from build123d import *

# Parameters (mm, degrees)
F0_W     = 75
F0_H     = 75
F0_R     = 3.75
F1_DEPTH = 2
F2_DEPTH = 16
F3_W     = 75
F3_H     = 75
F3_R     = 3.75
F3_W_2   = 50
F3_H_2   = 50
F4_DEPTH = 6.5
F5_W     = 1
F5_H     = 1
F6_DEPTH = 1


with BuildPart() as f1:
    # F0 (on Top) → F1 (new body)
    with BuildSketch(Plane.XY):
        Rectangle(F0_W, F0_H)
        with Locations((-31.25, -31.25)):
            Circle(F0_R, mode=Mode.SUBTRACT)
        with Locations((31.25, -31.25)):
            Circle(F0_R, mode=Mode.SUBTRACT)
        with Locations((-31.25, 31.25)):
            Circle(F0_R, mode=Mode.SUBTRACT)
        with Locations((31.25, 31.25)):
            Circle(F0_R, mode=Mode.SUBTRACT)
        with Locations((-31.25, 31.25)):
            Circle(F0_R)
        with Locations((31.25, 31.25)):
            Circle(F0_R)
        with Locations((31.25, -31.25)):
            Circle(F0_R)
        with Locations((-31.25, -31.25)):
            Circle(F0_R)
    extrude(amount=F1_DEPTH)

    # F0 (on Top) → F2 (join)
    with BuildSketch(Plane.XY):
        with Locations((-31.25, -31.25)):
            Circle(F0_R)
        with Locations((31.25, -31.25)):
            Circle(F0_R)
        with Locations((-31.25, 31.25)):
            Circle(F0_R)
        with Locations((31.25, 31.25)):
            Circle(F0_R)
    extrude(amount=F2_DEPTH)

    # F3 (on face) → F4 (join)
    with BuildSketch(Plane.XY.offset(2)):
        Rectangle(F3_W, F3_H)
        with Locations((-31.25, -31.25)):
            Circle(F3_R, mode=Mode.SUBTRACT)
        with Locations((31.25, -31.25)):
            Circle(F3_R, mode=Mode.SUBTRACT)
        with Locations((-31.25, 31.25)):
            Circle(F3_R, mode=Mode.SUBTRACT)
        Rectangle(F3_W_2, F3_H_2, mode=Mode.SUBTRACT)
        with Locations((31.25, 31.25)):
            Circle(F3_R, mode=Mode.SUBTRACT)
    extrude(amount=F4_DEPTH)

    # F5 (on face) → F6 (cut)
    with BuildSketch(Plane.XY):
        with BuildLine():
            Line((-32.5, -34.7855339059), (-32.5, -37.5))
            Line((-32.5, -37.5), (-31.5, -37.5))
            Line((-31.5, -37.5), (-31.5, -34.9916573868))
            ThreePointArc((-31.5, -34.9916573868), (-32.0070480317, -34.9227888964), (-32.5, -34.7855339059))
        make_face()
        with BuildLine():
            Line((-32.5, -32.5), (-32.5, -34.7855339059))
            ThreePointArc((-32.5, -34.7855339059), (-32.0070480317, -34.9227888964), (-31.5, -34.9916573868))
            Line((-31.5, -34.9916573868), (-31.5, -32.5))
            Line((-31.5, -32.5), (-32.5, -32.5))
        make_face()
        with BuildLine():
            Line((31.5, -34.9916573868), (31.5, -37.5))
            Line((31.5, -37.5), (32.5, -37.5))
            Line((32.5, -37.5), (32.5, -34.7855339059))
            ThreePointArc((32.5, -34.7855339059), (32.0070480317, -34.9227888964), (31.5, -34.9916573868))
        make_face()
        with BuildLine():
            Line((-34.7855339059, -32.5), (-32.5, -32.5))
            Line((-32.5, -32.5), (-32.5, -31.5))
            Line((-32.5, -31.5), (-34.9916573868, -31.5))
            ThreePointArc((-34.9916573868, -31.5), (-34.9227888964, -32.0070480317), (-34.7855339059, -32.5))
        make_face()
        with Locations((-32, -32)):
            Rectangle(F5_W, F5_H)
        with BuildLine():
            Line((-37.5, -32.5), (-34.7855339059, -32.5))
            ThreePointArc((-34.7855339059, -32.5), (-34.9227888964, -32.0070480317), (-34.9916573868, -31.5))
            Line((-34.9916573868, -31.5), (-37.5, -31.5))
            Line((-37.5, -31.5), (-37.5, -32.5))
        make_face()
        with BuildLine():
            Line((-31.5, -31.5), (-31.5, -32.5))
            Line((-31.5, -32.5), (-27.7144660941, -32.5))
            ThreePointArc((-27.7144660941, -32.5), (-27.5772111036, -32.0070480317), (-27.5083426132, -31.5))
            Line((-27.5083426132, -31.5), (-31.5, -31.5))
        make_face()
        with BuildLine():
            ThreePointArc((-27.5083426132, -31.5), (-27.5772111036, -32.0070480317), (-27.7144660941, -32.5))
            Line((-27.7144660941, -32.5), (27.7144660941, -32.5))
            ThreePointArc((27.7144660941, -32.5), (27.5772111036, -32.0070480317), (27.5083426132, -31.5))
            Line((27.5083426132, -31.5), (-27.5083426132, -31.5))
        make_face()
        with BuildLine():
            Line((31.5, -32.5), (31.5, -34.9916573868))
            ThreePointArc((31.5, -34.9916573868), (32.0070480317, -34.9227888964), (32.5, -34.7855339059))
            Line((32.5, -34.7855339059), (32.5, -32.5))
            Line((32.5, -32.5), (31.5, -32.5))
        make_face()
        with BuildLine():
            Line((-32.5, -27.7144660941), (-32.5, -31.5))
            Line((-32.5, -31.5), (-31.5, -31.5))
            Line((-31.5, -31.5), (-31.5, -27.5083426132))
            ThreePointArc((-31.5, -27.5083426132), (-32.0070480317, -27.5772111036), (-32.5, -27.7144660941))
        make_face()
        with BuildLine():
            ThreePointArc((27.5083426132, -31.5), (27.5772111036, -32.0070480317), (27.7144660941, -32.5))
            Line((27.7144660941, -32.5), (31.5, -32.5))
            Line((31.5, -32.5), (31.5, -31.5))
            Line((31.5, -31.5), (27.5083426132, -31.5))
        make_face()
        with Locations((32, -32)):
            Rectangle(F5_W, F5_H)
        with BuildLine():
            Line((-32.5, 27.7144660941), (-32.5, -27.7144660941))
            ThreePointArc((-32.5, -27.7144660941), (-32.0070480317, -27.5772111036), (-31.5, -27.5083426132))
            Line((-31.5, -27.5083426132), (-31.5, 27.5083426132))
            ThreePointArc((-31.5, 27.5083426132), (-32.0070480317, 27.5772111036), (-32.5, 27.7144660941))
        make_face()
        with BuildLine():
            Line((-37.5, 32.5), (-37.5, 31.5))
            Line((-37.5, 31.5), (-34.9916573868, 31.5))
            ThreePointArc((-34.9916573868, 31.5), (-34.9227888964, 32.0070480317), (-34.7855339059, 32.5))
            Line((-34.7855339059, 32.5), (-37.5, 32.5))
        make_face()
        with BuildLine():
            Line((32.5, -31.5), (32.5, -32.5))
            Line((32.5, -32.5), (34.7855339059, -32.5))
            ThreePointArc((34.7855339059, -32.5), (34.9227888964, -32.0070480317), (34.9916573868, -31.5))
            Line((34.9916573868, -31.5), (32.5, -31.5))
        make_face()
        with BuildLine():
            ThreePointArc((34.9916573868, -31.5), (34.9227888964, -32.0070480317), (34.7855339059, -32.5))
            Line((34.7855339059, -32.5), (37.5, -32.5))
            Line((37.5, -32.5), (37.5, -31.5))
            Line((37.5, -31.5), (34.9916573868, -31.5))
        make_face()
        with BuildLine():
            Line((31.5, -27.5083426132), (31.5, -31.5))
            Line((31.5, -31.5), (32.5, -31.5))
            Line((32.5, -31.5), (32.5, -27.7144660941))
            ThreePointArc((32.5, -27.7144660941), (32.0070480317, -27.5772111036), (31.5, -27.5083426132))
        make_face()
        with BuildLine():
            Line((-32.5, 31.5), (-32.5, 27.7144660941))
            ThreePointArc((-32.5, 27.7144660941), (-32.0070480317, 27.5772111036), (-31.5, 27.5083426132))
            Line((-31.5, 27.5083426132), (-31.5, 31.5))
            Line((-31.5, 31.5), (-32.5, 31.5))
        make_face()
        with BuildLine():
            ThreePointArc((-34.7855339059, 32.5), (-34.9227888964, 32.0070480317), (-34.9916573868, 31.5))
            Line((-34.9916573868, 31.5), (-32.5, 31.5))
            Line((-32.5, 31.5), (-32.5, 32.5))
            Line((-32.5, 32.5), (-34.7855339059, 32.5))
        make_face()
        with BuildLine():
            Line((31.5, 27.5083426132), (31.5, -27.5083426132))
            ThreePointArc((31.5, -27.5083426132), (32.0070480317, -27.5772111036), (32.5, -27.7144660941))
            Line((32.5, -27.7144660941), (32.5, 27.7144660941))
            ThreePointArc((32.5, 27.7144660941), (32.0070480317, 27.5772111036), (31.5, 27.5083426132))
        make_face()
        with Locations((-32, 32)):
            Rectangle(F5_W, F5_H)
        with BuildLine():
            Line((-31.5, 32.5), (-31.5, 31.5))
            Line((-31.5, 31.5), (-27.5083426132, 31.5))
            ThreePointArc((-27.5083426132, 31.5), (-27.5772111036, 32.0070480317), (-27.7144660941, 32.5))
            Line((-27.7144660941, 32.5), (-31.5, 32.5))
        make_face()
        with BuildLine():
            Line((31.5, 31.5), (31.5, 27.5083426132))
            ThreePointArc((31.5, 27.5083426132), (32.0070480317, 27.5772111036), (32.5, 27.7144660941))
            Line((32.5, 27.7144660941), (32.5, 31.5))
            Line((32.5, 31.5), (31.5, 31.5))
        make_face()
        with BuildLine():
            Line((34.9916573868, 31.5), (37.5, 31.5))
            Line((37.5, 31.5), (37.5, 32.5))
            Line((37.5, 32.5), (34.7855339059, 32.5))
            ThreePointArc((34.7855339059, 32.5), (34.9227888964, 32.0070480317), (34.9916573868, 31.5))
        make_face()
        with BuildLine():
            Line((-32.5, 34.7855339059), (-32.5, 32.5))
            Line((-32.5, 32.5), (-31.5, 32.5))
            Line((-31.5, 32.5), (-31.5, 34.9916573868))
            ThreePointArc((-31.5, 34.9916573868), (-32.0070480317, 34.9227888964), (-32.5, 34.7855339059))
        make_face()
        with BuildLine():
            Line((-32.5, 37.5), (-32.5, 34.7855339059))
            ThreePointArc((-32.5, 34.7855339059), (-32.0070480317, 34.9227888964), (-31.5, 34.9916573868))
            Line((-31.5, 34.9916573868), (-31.5, 37.5))
            Line((-31.5, 37.5), (-32.5, 37.5))
        make_face()
        with BuildLine():
            ThreePointArc((-27.7144660941, 32.5), (-27.5772111036, 32.0070480317), (-27.5083426132, 31.5))
            Line((-27.5083426132, 31.5), (27.5083426132, 31.5))
            ThreePointArc((27.5083426132, 31.5), (27.5772111036, 32.0070480317), (27.7144660941, 32.5))
            Line((27.7144660941, 32.5), (-27.7144660941, 32.5))
        make_face()
        with BuildLine():
            Line((27.5083426132, 31.5), (31.5, 31.5))
            Line((31.5, 31.5), (31.5, 32.5))
            Line((31.5, 32.5), (27.7144660941, 32.5))
            ThreePointArc((27.7144660941, 32.5), (27.5772111036, 32.0070480317), (27.5083426132, 31.5))
        make_face()
        with Locations((32, 32)):
            Rectangle(F5_W, F5_H)
        with BuildLine():
            Line((32.5, 31.5), (34.9916573868, 31.5))
            ThreePointArc((34.9916573868, 31.5), (34.9227888964, 32.0070480317), (34.7855339059, 32.5))
            Line((34.7855339059, 32.5), (32.5, 32.5))
            Line((32.5, 32.5), (32.5, 31.5))
        make_face()
        with BuildLine():
            Line((31.5, 34.9916573868), (31.5, 32.5))
            Line((31.5, 32.5), (32.5, 32.5))
            Line((32.5, 32.5), (32.5, 34.7855339059))
            ThreePointArc((32.5, 34.7855339059), (32.0070480317, 34.9227888964), (31.5, 34.9916573868))
        make_face()
        with BuildLine():
            Line((32.5, 37.5), (31.5, 37.5))
            Line((31.5, 37.5), (31.5, 34.9916573868))
            ThreePointArc((31.5, 34.9916573868), (32.0070480317, 34.9227888964), (32.5, 34.7855339059))
            Line((32.5, 34.7855339059), (32.5, 37.5))
        make_face()
    extrude(amount=F6_DEPTH, mode=Mode.SUBTRACT)


solid = f1.part
Can you work these out from the model? Positions are in its coordinate system, mm. A direction names the side the tool comes from. Coordinates: 2 decimals unless noted, no trailing zeros. Order: outer loops, then holes, each group sorted by start corner. A loop starts at its lowest first (then second) coordinate and runs counter-clockwise, first axis right, second up. Notation, with made-up numbers: M 1.5,41 L 52.5,41 A33 cw 52.5,73 Z; hole C 57,52 d8. An arc over 180 degrees is marked long. Write item = value, one per line.
(1) For faces 1 (the face through (0, 0, 2)), 2 (the face through (0, -35, 0)), which set-ups out of +Z, -Z, +X, -X, +Y, -Y let a thin tool reach every point of the face, with its end or its side?
Results are:
face_1 = +Z
face_2 = -Z, +X, -X, +Y, -Y
(2) Suppose I cut it at D-D on z = 15. Please give me the cut outline in (x, y).
Results are:
outline = C -31.25,-31.25 d7.5; C -31.25,31.25 d7.5; C 31.25,-31.25 d7.5; C 31.25,31.25 d7.5
(3) I need wall thicknesses on line 1 along Y through (x, z) = (1, 5.25); line 2 along Z through (x, y) = (10, -22.5). Which ranges of each line are inside material? Lowest first, please. Write a range as [from, to].
Results are:
line_1 = [-37.5, -25], [25, 37.5]
line_2 = [0, 2]
(4) Suppose I cut it at A-A on z = 3.5. Please give me the cut outline in (x, y), plus the area to 4 significant figures.
Results are:
outline = M -37.5,-37.5 L 37.5,-37.5 L 37.5,37.5 L -37.5,37.5 Z; hole M -25,-25 L 25,-25 L 25,25 L -25,25 Z
area = 3,125 mm2
(5) If we mould it in two halves opening along Y, with no side actions, what happens to faces 3 (the face through (0, 25, 5)), 4 (the face through (35, 0, 0))? For each: pulls with the +Y half, pulls with the -Y half, needs draft (parallel to the pull), parting line crosses it, or undercut.
Results are:
face_3 = undercut
face_4 = needs draft
(6) Suppose I cut it at B-B on x = 22. Please give me the cut outline in (y, z), plus the area to 4 significant figures.
Results are:
outline = M -37.5,0 L -32.5,0 L -32.5,1 L -31.5,1 L -31.5,0 L 31.5,0 L 31.5,1 L 32.5,1 L 32.5,0 L 37.5,0 L 37.5,8.5 L 25,8.5 L 25,2 L -25,2 L -25,8.5 L -37.5,8.5 Z
area = 310.5 mm2
(7) For pin 1 Ø12 at (x, y) = (-2, 18) entering from -Z; pin 2 Ø6 at (x, y) = (20, 6.5) entering from +Z, each with a flat end and sliding along its axis, tell me the tip position at first contact or that it passes through.
Results are:
pin_1 = 0
pin_2 = 2
